Build history of the part. All positions in model axes, mm. Give positions to 0.01 mm unless a question says otherwise; leave off trailing zeros. Loops run counter-clockwise (first coordinate to the right, second up) from the corner with the lowest first, then second, coordinate; pieces in that order, holes last. Notation, with made-up numbers: M 6,-34 L 38,-34 A21 ccw 38,-2 Z; hole C -2.75,51 d9. An arc over 180 degrees is marked long. Put each result on its own line as item: value.
Autodesk Inventor part; units mm, degrees
ref_plane "YZ Plane" through (0, 0, 0) normal (1, 0, 0) x (0, 1, 0)
ref_plane "XZ Plane" through (0, 0, 0) normal (0, 1, 0) x (-1, 0, 0)
ref_plane "XY Plane" through (0, 0, 0) normal (0, 0, 1) x (1, 0, 0)
sketch "Sketch1" plane through (0, 0, 0) normal (1, 0, 0) x (0, 1, 0)
  line L0 (0, 0) -> (25.4, 0)
  line L1 (25.4, 0) -> (25.4, -127)
  line L2 (25.4, -127) -> (0, -127)
  line L3 (0, -127) -> (0, 0)
  line L4 (101.6, -50.8) -> (25.4, -50.8)
  line L5 (25.4, -50.8) -> (25.4, -76.2)
  line L6 (25.4, -76.2) -> (101.6, -76.2)
  line L7 (101.6, -76.2) -> (101.6, -50.8)
  circle A0 centre (12.7, -25.4) radius 2.5527
  circle A1 centre (12.7, -50.8) radius 2.5527
  circle A2 centre (12.7, -76.2) radius 2.5527
  circle A3 centre (12.7, -101.6) radius 2.5527
  circle A4 centre (88.9, -63.5) radius 2.5527
  circle A5 centre (63.5, -63.5) radius 2.5527
  circle A6 centre (38.1, -63.5) radius 2.5527
  line L8 (25.4, 0) -> (101.6, -50.8)
  line L9 (101.6, -76.2) -> (25.4, -127)
  point P0 (25.4, -63.5)
  dimension "d0" = 25.4
  dimension "d1" = 127
  dimension "d2" = 76.2
  dimension "d3" = 25.4
  dimension "d4" = 5.1054
  dimension "d5" = 25.4
  dimension "d6" = 12.7
  dimension "d9" = 25.4
  dimension "d14" = 5.1054
  dimension "d15" = 12.7
  dimension "d16" = 12.7
  dimension "d19" = 25.4
extrude "Extrusion1" add sketch "Sketch1" along normal blind 3.175
properties part number "T-Gusset" material "Aluminum 6061"
Q1. Probe line 1 (Z direction, x = 2.05, y = 12.7); line 2 (Z direction, x = 2.65, y = 14); line 3 (Y direction, x = 1, z = -102). List the from-to ranges inside material, lowest first. Write a range as from..to.
Here are the results:
line 1: -127..-104.15, -99.05..-78.75, -73.65..-53.35, -48.25..-27.95, -22.85..0
line 2: -127..-103.8, -99.4..-78.4, -74..-53, -48.6..-27.6, -23.2..0
line 3: 0..10.18, 15.22..62.9
Q2. Slice it at C-C (x = 1.6). List the corners of the cut face in (y, z).
Here are the results:
outline: M 0,-127 L 25.4,-127 L 101.6,-76.2 L 101.6,-50.8 L 25.4,0 L 0,0 Z; hole C 12.7,-101.6 d5.11; hole C 12.7,-76.2 d5.11; hole C 12.7,-50.8 d5.11; hole C 12.7,-25.4 d5.11; hole C 38.1,-63.5 d5.11; hole C 63.5,-63.5 d5.11; hole C 88.9,-63.5 d5.11
Q3. Slice it at D-D (y = 63.5). List the corners of the cut face in (x, z) (3 decimals).
Here are the results:
outline: M 0,-101.6 L 3.175,-101.6 L 3.175,-66.053 L 0,-66.053 Z; M 0,-60.947 L 3.175,-60.947 L 3.175,-25.4 L 0,-25.4 Z
Q4. Slice it at A-A (z = -101.6). List the corners of the cut face in (x, y) (3 decimals).
Here are the results:
outline: M 0,0 L 3.175,0 L 3.175,10.147 L 0,10.147 Z; M 0,15.253 L 3.175,15.253 L 3.175,63.5 L 0,63.5 Z
Q5. Drop flat-ended pins along their axis: pin 1 Ø1.5 at (x, y) = (0.5, 81) entering from +Z; pin 2 Ø1.5 at (x, z) = (1, -106.5) entering from -Y. Give the stop position or say it passes through.
Here are the results:
pin 1: z = -36.57
pin 2: y = 0
Q6. Mould opens along Y. For faces 1 (the flat face through (1.565, 62.967, -25.044)), 2 (the flat face through (0, 50, -63)), 3 (the cylindrical face through (1.565, 37.547, -61.008)) say: pulls with the +Y half, pulls with the -Y half, needs draft (parallel to the pull), parting line crosses it, or undercut.
Here are the results:
face 1: pulls with the +Y half
face 2: needs draft
face 3: undercut
Q7. Slice it at B-B (z = -63.5). List the corners of the cut face in (x, y) (3 decimals), and give its area (3 significant figures).
Here are the results:
outline: M 0,0 L 3.175,0 L 3.175,35.547 L 0,35.547 Z; M 0,40.653 L 3.175,40.653 L 3.175,60.947 L 0,60.947 Z; M 0,66.053 L 3.175,66.053 L 3.175,86.347 L 0,86.347 Z; M 0,91.453 L 3.175,91.453 L 3.175,101.6 L 0,101.6 Z
area: 274 mm²
